```python
from build123d import *

# Parameters (mm, degrees)
BOSS_EXTRUDE1_DEPTH = 20
SKETCH3_R           = 10
SKETCH3_R_2         = 7
SKETCH3_R_3         = 5
CUT_EXTRUDE1_DEPTH  = 102.044544633


with BuildPart() as part:
    # Sketch2 → Boss-Extrude1 (new body)
    with BuildSketch(Plane.XY):
        with BuildLine():
            ThreePointArc((32.82507564, 3.393288852), (30.919385889, 11.532197372), (27.029816197, 18.931165741))
            ThreePointArc((27.029816197, 18.931165741), (17.392020832, 40.004906757), (15.890255583, 63.129230769))
            ThreePointArc((15.890255583, 63.129230769), (0, 81), (-15.890255583, 63.129230769))
            ThreePointArc((-15.890255583, 63.129230769), (-17.392020832, 40.004906757), (-27.029816197, 18.931165741))
            ThreePointArc((-27.029816197, 18.931165741), (-30.919385889, 11.532197372), (-32.82507564, 3.393288852))
            ThreePointArc((-32.82507564, 3.393288852), (-37.963155814, -8.050663767), (-48.906353625, -14.183390817))
            ThreePointArc((-48.906353625, -14.183390817), (-56.22107819, -27.869330305), (-41.330511904, -32.237530257))
            ThreePointArc((-41.330511904, -32.237530257), (-20.895992582, -30.900485472), (-9.997178571, -48.237530257))
            ThreePointArc((-9.997178571, -48.237530257), (0, -58), (9.997178571, -48.237530257))
            ThreePointArc((9.997178571, -48.237530257), (20.895992582, -30.900485472), (41.330511904, -32.237530257))
            ThreePointArc((41.330511904, -32.237530257), (56.22107819, -27.869330305), (48.906353625, -14.183390817))
            ThreePointArc((48.906353625, -14.183390817), (37.963155814, -8.050663767), (32.82507564, 3.393288852))
        make_face()
    extrude(amount=-BOSS_EXTRUDE1_DEPTH)

    # Sketch3 → Cut-Extrude1 (cut, through all)
    with BuildSketch(Plane(origin=(0, 0, -20), x_dir=(-1, 0, 0), z_dir=(0, 0, -1))):
        with Locations((0, 65)):
            Circle(SKETCH3_R)
        with Locations((47, -24)):
            Circle(SKETCH3_R_2)
        with Locations((0, -48)):
            Circle(SKETCH3_R_3)
        with Locations((-47, -24)):
            Circle(SKETCH3_R_2)
        with BuildLine():
            ThreePointArc((-14.687363137, 13.575027222), (-17.320508076, 10), (-19.1, 5.93211598))
            ThreePointArc((-19.1, 5.93211598), (-14, 0), (-19.1, -5.93211598))
            ThreePointArc((-19.1, -5.93211598), (-17.320508076, -10), (-14.687363137, -13.575027222))
            ThreePointArc((-14.687363137, -13.575027222), (-7, -12.124355653), (-4.412636863, -19.507143202))
            ThreePointArc((-4.412636863, -19.507143202), (0, -20), (4.412636863, -19.507143202))
            ThreePointArc((4.412636863, -19.507143202), (7, -12.124355653), (14.687363137, -13.575027222))
            ThreePointArc((14.687363137, -13.575027222), (17.320508076, -10), (19.1, -5.93211598))
            ThreePointArc((19.1, -5.93211598), (14, 0), (19.1, 5.93211598))
            ThreePointArc((19.1, 5.93211598), (17.320508076, 10), (14.687363137, 13.575027222))
            ThreePointArc((14.687363137, 13.575027222), (7, 12.124355653), (4.412636863, 19.507143202))
            ThreePointArc((4.412636863, 19.507143202), (0, 20), (-4.412636863, 19.507143202))
            ThreePointArc((-4.412636863, 19.507143202), (-7, 12.124355653), (-14.687363137, 13.575027222))
        make_face()
    extrude(amount=-CUT_EXTRUDE1_DEPTH, mode=Mode.SUBTRACT)


solid = part.part
```
Here's how the part is built. I have some questions about the finished solid (model axes, mm). Coordinates: 2 decimals unless noted, no trailing zeros. Order: outer loops, then holes, each group sorted by start corner. A loop starts at its lowest first (then second) coordinate and runs counter-clockwise, first axis right, second up.
Item 1: If we section it at B-B, the plane x = 0: List the corners of the cut face in (y, z) for me, then the cut area to 3 significant figures.
Response values:
outline: (-58, -20) - (-53, -20) - (-53, 0) - (-58, 0) - close; (-43, -20) - (-20, -20) - (-20, 0) - (-43, 0) - close; (20, -20) - (55, -20) - (55, 0) - (20, 0) - close; (75, -20) - (81, -20) - (81, 0) - (75, 0) - close
area: 1,380 mm2
Item 2: If we section it at C-C, the plane y = -24: List the corners of the cut face in (x, z) for me.
Response values:
outline: (-57, -20) - (-54, -20) - (-54, 0) - (-57, 0) - close; (-40, -20) - (40, -20) - (40, 0) - (-40, 0) - close; (54, -20) - (57, -20) - (57, 0) - (54, 0) - close
Item 3: Thinking about a two-plate mould opening in Y: for faces 1 (the face through (12, 12, -20)), 2 (the face through (56.12, -28.1, -9.86)), 3 (the face through (0, 20, -10)), which applies, pulls with the +Y half, pulls with the -Y half, needs draft (parallel to the pull), parting line crosses it, or undercut?
Response values:
face 1: needs draft
face 2: parting line crosses it
face 3: undercut
Item 4: I'm going to push flat-ended pins straight in: pin 1 Ø4 at (y, z) = (22.5, -15) entering from +X; pin 2 Ø6 at (y, z) = (55.5, -14) entering from -X; pin 3 Ø12.5 at (x, y) = (47, -24) entering from +Z; pin 4 Ø5 at (x, z) = (-12, -12) entering from +Y. Where does each tip first touch, or does it pass through?
Response values:
pin 1: stops at x = 25.97
pin 2: stops at x = -15.53
pin 3: passes through
pin 4: stops at y = 77.87
Item 5: If we section it at A-A, the plane y = 65: List the corners of the cut face in (x, z) for me.
Response values:
outline: (-16, -20) - (-10, -20) - (-10, 0) - (-16, 0) - close; (10, -20) - (16, -20) - (16, 0) - (10, 0) - close
Item 6: If we section it at D-D, the plane z = -3: List the corners of the cut face in (x, y) for me, then the cut area to 3 significant figures.
Response values:
outline: (-48.91, -14.18) arc R10 ccw (long way) to (-41.33, -32.24) arc R20 cw to (-10, -48.24) arc R10 ccw to (10, -48.24) arc R20 cw to (41.33, -32.24) arc R10 ccw (long way) to (48.91, -14.18) arc R20 cw to (32.83, 3.39) arc R33 ccw to (27.03, 18.93) arc R64 cw to (15.89, 63.13) arc R16 ccw (long way) to (-15.89, 63.13) arc R64 cw to (-27.03, 18.93) arc R33 ccw to (-32.83, 3.39) arc R20 cw to start; hole circle Ø14 at (-47, -24); hole (-19.1, -5.93) arc R20 ccw to (-14.69, -13.58) arc R6 cw to (-4.41, -19.51) arc R20 ccw to (4.41, -19.51) arc R6 cw to (14.69, -13.58) arc R20 ccw to (19.1, -5.93) arc R6 cw to (19.1, 5.93) arc R20 ccw to (14.69, 13.58) arc R6 cw to (4.41, 19.51) arc R20 ccw to (-4.41, 19.51) arc R6 cw to (-14.69, 13.58) arc R20 ccw to (-19.1, 5.93) arc R6 cw to start; hole circle Ø20 at (0, 65); hole circle Ø10 at (0, -48); hole circle Ø14 at (47, -24)
area: 5,200 mm2
Item 7: I need wall thicknesses on probe 1 along Y at (x, z) = (8.5, -3); probe 2 along Y at (x, z) = (-7, -3); probe 3 along X at (y, z) = (-25, -8.25). Which ranges of each line are inside material? Lowest first, please.
Response values:
probe 1: y = -53.27 to -11.51, 11.51 to 59.73, 70.27 to 78.56
probe 2: y = -55.14 to -12.12, 12.12 to 57.86, 72.14 to 79.39
probe 3: x = -56.95 to -53.93, -40.07 to 40.07, 53.93 to 56.95
